Can you work these out from the drawing? Everything is in mm from the part's minimum corner. Give positions to 0.01 mm unless a question says otherwise; leave off trailing zeros. Return JSON: item names as keys, results as strings.
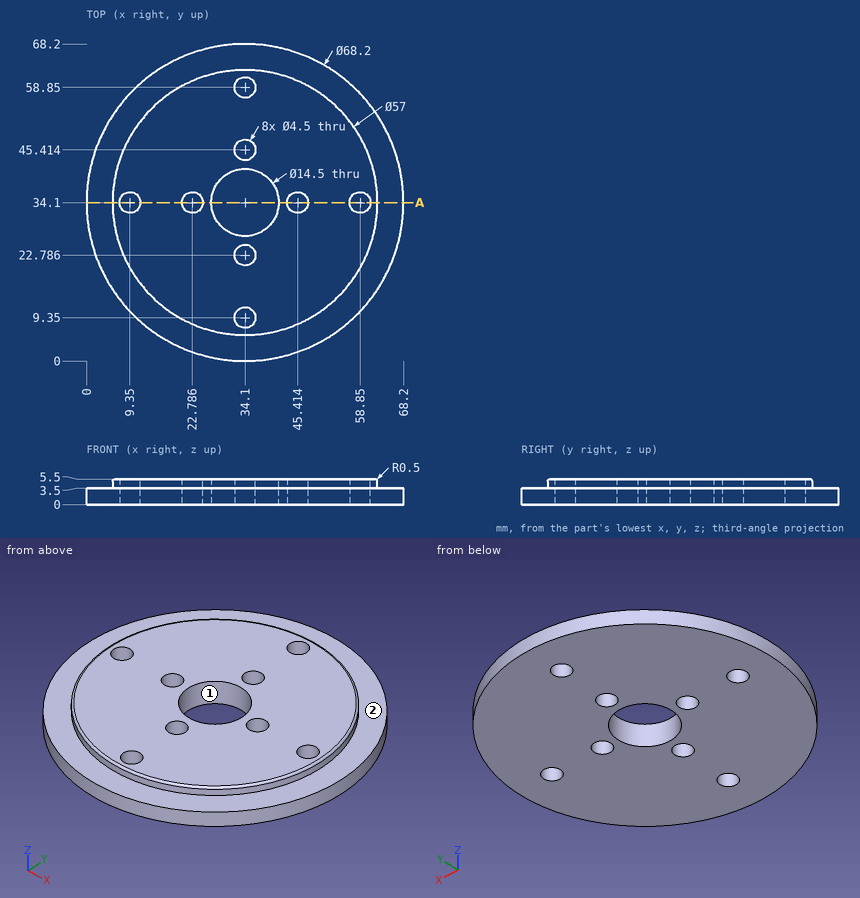
1. Suppose I cut it at A-A, the plane y = 34.1. Count the separate pieces of the cut face and the enclosed holes in it, and give its area (3 significant figures).
Taken from the geometry:
{"separate pieces": "6", "enclosed holes": "0", "area": "174 mm²"}
2. If we mould it in two halves opening along X, with no side actions, what happens to the marked faces 1 and 2? For each: released by +X, released by -X, zero draft, split by the parting line, or undercut.
Taken from the geometry:
{"face 1": "undercut", "face 2": "zero draft"}
3. If I drill on line 1 (Y direction, x = 34.1, z = 1.55); line 2 (Z direction, x = 64.5, y = 46); line 3 (Y direction, x = 9.35, z = 2.05), over which ranges is the centre line in solid material (lowest first)? Write a range as [from, to].
Taken from the geometry:
{"line 1": "y = [0, 7.1], [11.6, 20.54], [25.04, 26.85], [41.35, 43.16], [47.66, 56.6], [61.1, 68.2]", "line 2": "z = [0, 3.5]", "line 3": "y = [10.64, 31.85], [36.35, 57.56]"}
4. For pin 1 Ø2.5 at (x, y) = (22.79, 34.1) entering from -Z, with a flat end and sliding along its axis, tell me the tip position at first contact or that it passes through.
Taken from the geometry:
{"pin 1": "passes through"}
